Geometry: final body of the model. Coordinates: model frame, mm. A direction names the side the tool comes from. Round coordinates to 2 decimals unless told otherwise and drop trailing zeros. Order: outer loops, then holes, each group sorted by start corner. A loop starts at its lowest first (then second) coordinate and runs counter-clockwise, first axis right, second up. Notation, with made-up numbers: (20, -28) - (39, -28) arc R25 cw to (39, 9) - close; hole circle Ø7 at (30, 59.5). An arc over 180 degrees is marked (long way). Put each result on its own line as item: value. Start each with the question number.
(1) Pull-direction query (X, two-part tool) for faces 1 (the face through (80, 175, 25.7)), 2 (the face through (70, 0, 15)), 3 (the face through (142, 98, 23)); classes: released by +X, released by -X, zero draft, split by the parting line, or undercut.
(2) Section C-C (z = 14). Output: boundary loops of the cut face in (x, y).
(3) Section A-A (x = 51). Output: boundary loops of the cut face in (y, z), and give its area (3 significant figures).
(4) Access query for faces 4 (the face through (115, 175, 28)), 5 (the face through (17, 67, 10)), 6 (the face through (142, 4.6, 18.5)), 7 (the face through (10.39, 89.76, 4.39)), 8 (the face through (30, 94, 23.7)). Directions: +Z, -Z, +X, -X, +Y, -Y. A direction counts if a zero-diameter tool reaches every point of the face in a straight line with its end or side. Return the directions, or none.
(5) Pin query (flat end, axial travel): P1, Ø4.5, axis at x = 161, y = 120, coming from the -Z side; P2, Ø11, axis at x = 154.5, z = 26.5, coming from the -Y side; P3, Ø1.7, axis at x = 65, y = 175, coming from the +Z side; P4, Ø4, axis at y = 145.5, z = 6.5, coming from the +X side. Return the tip coordinate at first contact, or that it passes through.
(6) Section B-B (y = 111). Output: boundary loops of the cut face in (x, z), and give its area (3 significant figures).
(7) Material intervals for L1, parallel to Y at x = 161, z = 27.8; L2, parallel to X at y = 175, z = 24.3; L3, parallel to X at y = 175, z = 22, sorted ascending. Write a range as [from, to].
(8) Section D-D (y = 143). Output: boundary loops of the cut face in (x, z).
from build123d import *

# Parameters (mm, degrees)
CROQUIS1_W              = 180
CROQUIS1_H              = 180
SALIENTE_EXTRUIR1_DEPTH = 30.7
CROQUIS2_W              = 162.21
CROQUIS2_H              = 162.99
CORTAR_EXTRUIR1_DEPTH   = 20.7
CROQUIS4_W              = 175
CROQUIS4_H              = 10.7
CORTAR_EXTRUIR2_DEPTH   = 175
CORTAR_EXTRUIR3_REACH   = 258.403
CROQUIS5_W              = 38
CROQUIS5_H              = 30.7
CROQUIS6_W              = 38
CROQUIS6_H              = 82.99
CORTAR_EXTRUIR4_DEPTH   = 5
CROQUIS7_W              = 50
CROQUIS7_H              = 175
CORTAR_EXTRUIR5_DEPTH   = 3
CROQUIS8_W              = 70
CROQUIS8_H              = 10
CORTAR_EXTRUIR6_DEPTH   = 5
CHAFL_N1_SIZE           = 15
CHAFL_N1_SIZE2          = 8.660254038
CROQUIS9_R              = 1.4
CORTAR_EXTRUIR7_DEPTH   = 20


with BuildPart() as part:
    # Croquis1 → Saliente-Extruir1 (new body)
    with BuildSketch(Plane.XY):
        with Locations((90, 90)):
            Rectangle(CROQUIS1_W, CROQUIS1_H)
    extrude(amount=SALIENTE_EXTRUIR1_DEPTH)

    # Croquis2 → Cortar-Extruir1 (cut)
    with BuildSketch(Plane(origin=(0, 0, 0), x_dir=(-1, 0, 0), z_dir=(0, 0, -1))):
        with Locations((-98.895, 98.505)):
            Rectangle(CROQUIS2_W, CROQUIS2_H)
    extrude(amount=-CORTAR_EXTRUIR1_DEPTH, mode=Mode.SUBTRACT)

    # Croquis4 → Cortar-Extruir2 (cut)
    with BuildSketch(Plane(origin=(0, 180, 0), x_dir=(1, 0, 0), z_dir=(0, 1, 0))):
        with Locations((92.5, -15.35)):
            Rectangle(CROQUIS4_W, CROQUIS4_H)
    extrude(amount=-CORTAR_EXTRUIR2_DEPTH, mode=Mode.SUBTRACT)

    # Cortar-Extruir3: up to this face of the body (flat: up to its plane)
    cortar_extruir3_end = Plane(part.part.faces().sort_by_distance((98.895, 17.01, 5))[0])
    # Croquis5 → Cortar-Extruir3 (cut, up to the picked face)
    with BuildSketch(Plane.XZ, mode=Mode.PRIVATE) as cortar_extruir3_sk1:
        with Locations((161, 15.35)):
            Rectangle(CROQUIS5_W, CROQUIS5_H)
    cortar_extruir3_tool1 = split(extrude(cortar_extruir3_sk1.sketch, amount=-CORTAR_EXTRUIR3_REACH, mode=Mode.PRIVATE), bisect_by=cortar_extruir3_end, keep=Keep.BOTH, mode=Mode.PRIVATE)
    add(cortar_extruir3_tool1.solids().sort_by(Axis((161, 0, 15.35), (0, 1, 0)))[0], mode=Mode.SUBTRACT)

    # Croquis6 → Cortar-Extruir4 (cut)
    with BuildSketch(Plane(origin=(0, 0, 20.7), x_dir=(-1, 0, 0), z_dir=(0, 0, -1))):
        with Locations((-161, 98.505)):
            Rectangle(CROQUIS6_W, CROQUIS6_H)
    extrude(amount=-CORTAR_EXTRUIR4_DEPTH, mode=Mode.SUBTRACT)

    # Croquis7 → Cortar-Extruir5 (cut)
    with BuildSketch(Plane(origin=(0, 0, 20.7), x_dir=(-1, 0, 0), z_dir=(0, 0, -1))):
        with Locations((-30, 92.5)):
            Rectangle(CROQUIS7_W, CROQUIS7_H)
    extrude(amount=-CORTAR_EXTRUIR5_DEPTH, mode=Mode.SUBTRACT)

    # Croquis8 → Cortar-Extruir6 (cut)
    with BuildSketch(Plane.XY.offset(30.7)):
        with Locations((80, 175)):
            Rectangle(CROQUIS8_W, CROQUIS8_H)
    extrude(amount=-CORTAR_EXTRUIR6_DEPTH, mode=Mode.SUBTRACT)

    # Chaflán1
    chafl_n1_edges = [part.edges().sort_by_distance(p)[0] for p in [
        (17.79, 98.505, 0),
        (79.895, 17.01, 0),
    ]]
    chafl_n1_side = [part.faces().sort_by_distance(p)[0] for p in [
        (8.895, 177.707315983, 0),
    ]]
    chamfer(chafl_n1_edges, length=CHAFL_N1_SIZE, length2=CHAFL_N1_SIZE2, reference=chafl_n1_side[0])

    # Croquis9 → Cortar-Extruir7 (cut)
    with BuildSketch(Plane(origin=(0, 0, 20.7), x_dir=(-1, 0, 0), z_dir=(0, 0, -1))):
        with Locations((-161, 77.01)):
            Circle(CROQUIS9_R)
        with Locations((-161, 120)):
            Circle(CROQUIS9_R)
        with Locations((-65, 175)):
            Circle(CROQUIS9_R)
        with Locations((-95, 175)):
            Circle(CROQUIS9_R)
    extrude(amount=-CORTAR_EXTRUIR7_DEPTH, mode=Mode.SUBTRACT)


solid = part.part
Checks:
1. face 1: undercut
1. face 2: zero draft
1. face 3: released by +X
2. outline: (0, 0) - (142, 0) - (142, 5) - (5, 5) - (5, 180) - (0, 180) - close
3. outline: (0, 0) - (2.01, 0) - (17.01, 8.66) - (17.01, 10) - (5, 10) - (5, 23.7) - (180, 23.7) - (180, 25.7) - (170, 25.7) - (170, 30.7) - (0, 30.7) - close
3. area: 1,380 mm²
4. face 4: +Z, +Y
4. face 5: +X, +Y
4. face 6: +Z, -Z, +X, -Y
4. face 7: -Z, +X, +Y
4. face 8: +Y
5. P1: stops at z = 25.7
5. P2: stops at y = 17.01
5. P3: passes through
5. P4: stops at x = 17.51
6. outline: (0, 0) - (2.79, 0) - (17.79, 8.66) - (17.79, 10) - (5, 10) - (5, 23.7) - (55, 23.7) - (55, 20.7) - (142, 20.7) - (142, 25.7) - (180, 25.7) - (180, 30.7) - (0, 30.7) - close
6. area: 1,630 mm²
7. L1: y = [17.01, 75.61], [78.41, 118.6], [121.4, 180]
7. L2: x = [0, 63.6], [66.4, 93.6], [96.4, 180]
7. L3: x = [0, 5], [55, 63.6], [66.4, 93.6], [96.4, 180]
8. outline: (0, 0) - (2.79, 0) - (17.79, 8.66) - (17.79, 10) - (5, 10) - (5, 23.7) - (55, 23.7) - (55, 20.7) - (180, 20.7) - (180, 30.7) - (0, 30.7) - close
